Input: part model. Units: mm. Frame: model coordinates. Coordinates: 2 decimals unless noted, no trailing zeros. Write each loop counter-clockwise with the first axis right and the second up, starting at its lowest first coordinate (ties: lowest second). Pieces come first, ordered by that corner, then holes.
1) Section query A-A (y = 16.5). Output: boundary loops of the cut face in (x, z).
2) Section query C-C (z = -25). Output: boundary loops of the cut face in (x, y), then the cut area to 3 significant figures.
3) Section query D-D (x = 0.4). State how many separate pieces and enclosed holes the cut face has, then the cut area to 3 significant figures.
4) Pin query (flat end, axial travel): pin 1 Ø10 at (y, z) = (9.5, -5) entering from +X; pin 2 Ø1.5 at (x, z) = (0.5, -18.5) entering from +Y. Return the tip coordinate at first contact, or that it passes through.
5) Section query B-B (z = -6). Output: boundary loops of the cut face in (x, y).
6) Line query: L1, parallel to Z at x = 1.7, y = 15; L2, parallel to Y at x = 2.45, z = -7.5; L3, parallel to Y at x = 1.5, z = -10. Output: solid intervals per line, ascending.
from build123d import *

# Parameters (mm, degrees)
SKETCH1_R           = 1.872075336
SKETCH1_R_2         = 2
BOSS_EXTRUDE1_DEPTH = 2.5


with BuildPart() as part:
    # Sketch1 → Boss-Extrude1 (new body)
    with BuildSketch(Plane(origin=(0, 0, 0), x_dir=(0, 0, -1), z_dir=(1, 0, 0))):
        with BuildLine():
            Line((23.5, 7), (27, 7))
            ThreePointArc((27, 7), (30.535533906, 8.464466094), (32, 12))
            Line((32, 12), (32, 28.501))
            ThreePointArc((32, 28.501), (32.439046935, 29.560953065), (33.499, 30))
            Line((33.499, 30), (33.501, 30))
            ThreePointArc((33.501, 30), (34.560953065, 29.560953065), (35, 28.501))
            Line((35, 28.501), (35, 8))
            ThreePointArc((35, 8), (32.656854249, 2.343145751), (27, 0))
            Line((27, 0), (8, 0))
            ThreePointArc((8, 0), (2.343145751, 2.343145751), (0, 8))
            Line((0, 8), (0, 28.501))
            ThreePointArc((0, 28.501), (0.439046935, 29.560953065), (1.499, 30))
            Line((1.499, 30), (1.501, 30))
            ThreePointArc((1.501, 30), (2.560953065, 29.560953065), (3, 28.501))
            Line((3, 28.501), (3, 12))
            ThreePointArc((3, 12), (4.464466094, 8.464466094), (8, 7))
            Line((8, 7), (11.5, 7))
            ThreePointArc((11.5, 7), (12.914213562, 7.585786438), (13.5, 9))
            Line((13.5, 9), (13.5, 18))
            ThreePointArc((13.5, 18), (12, 19.5), (10.5, 18))
            Line((10.5, 18), (10.5, 11.49))
            ThreePointArc((10.5, 11.49), (9.917142495, 10.082857505), (8.51, 9.5))
            Line((8.51, 9.5), (8.49, 9.5))
            ThreePointArc((8.49, 9.5), (7.082857505, 10.082857505), (6.5, 11.49))
            Line((6.5, 11.49), (6.5, 25.01))
            ThreePointArc((6.5, 25.01), (7.082857505, 26.417142495), (8.49, 27))
            Line((8.49, 27), (26.51, 27))
            ThreePointArc((26.51, 27), (27.917142495, 26.417142495), (28.5, 25.01))
            Line((28.5, 25.01), (28.5, 11.49))
            ThreePointArc((28.5, 11.49), (27.917142495, 10.082857505), (26.51, 9.5))
            Line((26.51, 9.5), (26.49, 9.5))
            ThreePointArc((26.49, 9.5), (25.082857505, 10.082857505), (24.5, 11.49))
            Line((24.5, 11.49), (24.5, 18))
            ThreePointArc((24.5, 18), (23, 19.5), (21.5, 18))
            Line((21.5, 18), (21.5, 9))
            ThreePointArc((21.5, 9), (22.085786438, 7.585786438), (23.5, 7))
        make_face()
        with Locations((10, 23)):
            Circle(SKETCH1_R, mode=Mode.SUBTRACT)
        with Locations((25, 23)):
            Circle(SKETCH1_R, mode=Mode.SUBTRACT)
        with Locations((6, 4)):
            Circle(SKETCH1_R_2, mode=Mode.SUBTRACT)
        with Locations((29, 4)):
            Circle(SKETCH1_R_2, mode=Mode.SUBTRACT)
    extrude(amount=BOSS_EXTRUDE1_DEPTH)


solid = part.part
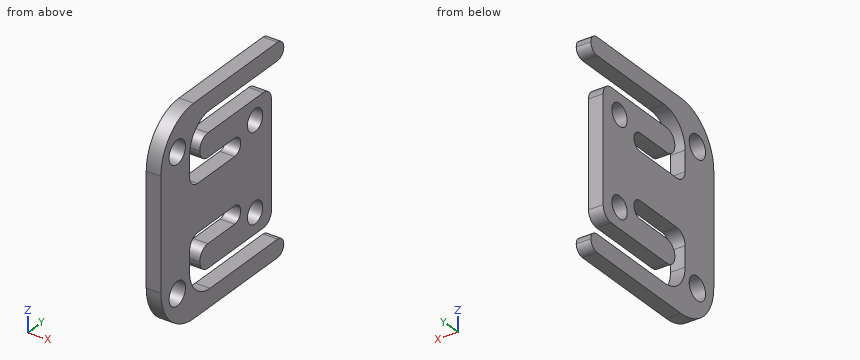
Answer:
1. outline: (0, -35) - (2.5, -35) - (2.5, -32) - (0, -32) - close; (0, -28.5) - (2.5, -28.5) - (2.5, -24.5) - (0, -24.5) - close; (0, -21.5) - (2.5, -21.5) - (2.5, -13.5) - (0, -13.5) - close; (0, -10.5) - (2.5, -10.5) - (2.5, -6.5) - (0, -6.5) - close; (0, -3) - (2.5, -3) - (2.5, 0) - (0, 0) - close
2. outline: (0, 0) - (2.5, 0) - (2.5, 7) - (0, 7) - close; (0, 10.17) - (2.5, 10.17) - (2.5, 21.13) - (0, 21.13) - close; (0, 24.87) - (2.5, 24.87) - (2.5, 27) - (0, 27) - close
2. area: 50.2 mm2
3. separate pieces: 1
3. enclosed holes: 4
3. area: 661 mm2
4. pin 1: stops at x = 2.5
4. pin 2: stops at y = 27
5. outline: (0, 0.25) - (2.5, 0.25) - (2.5, 2) - (0, 2) - close; (0, 6) - (2.5, 6) - (2.5, 7.42) - (0, 7.42) - close
6. L1: z = -35 to -32, -28.5 to -24.5, -21.5 to -13.5, -10.5 to -6.5, -3 to 0
6. L2: y = 0.02 to 2.68, 5.32 to 7.03, 9.76 to 26.74
6. L3: y = 0 to 7, 10.17 to 21.13, 24.87 to 27
